```python
from build123d import *

# Parameters (mm, degrees)
F0_R     = 20
F1_DEPTH = 6
F2_R     = 13.774889
F2_R_2   = 5.493426
F3_DEPTH = 2
F4_D     = 3


with BuildPart() as f1:
    # F0 (on Front) → F1 (new body)
    with BuildSketch(Plane.XZ):
        Circle(F0_R)
    extrude(amount=F1_DEPTH)

    # F2 (on face) → F3 (cut)
    with BuildSketch(Plane.XZ.offset(6)):
        Circle(F2_R)
        Circle(F2_R_2, mode=Mode.SUBTRACT)
    extrude(amount=-F3_DEPTH, mode=Mode.SUBTRACT)

    # F4 (through all)
    with Locations(Plane.XZ.offset(6)):
        with Locations((0, 0)):
            Hole(F4_D / 2)


solid = f1.part
```
Source: CAD feature listing. Evaluate the final solid. Frame: model axes, mm. A direction names the side the tool comes from. Give positions to 0.01 mm unless a question says otherwise; leave off trailing zeros. Loops run counter-clockwise (first coordinate to the right, second up) from the corner with the lowest first, then second, coordinate; pieces in that order, holes last. Notation, with made-up numbers: (48, -16) -> (84, -16) arc R12 ccw to (84, -3) -> close; hole circle Ø10 at (2, -37). An arc over 180 degrees is marked (long way). Put each result on its own line as item: value. Start each with the question number.
1) Material intervals for probe 1 along Z at (x, y) = (0, -4.8); probe 2 along X at (y, z) = (-4.15, -5); probe 3 along Y at (x, z) = (4, -13), sorted ascending.
2) Cut plane C-C (y = -5.25). Return loops of the section in (x, z).
3) Contact query for flat-ended pins moving along their axis: P1, Ø2, axis at x = 2, y = -1, coming from the +Z side (3 decimals); P2, Ø5, axis at x = -10.5, z = 6, coming from the -Y side; P3, Ø4, axis at x = 10, z = -4.5, coming from the -Y side. Output: stop coordinate, or through.
4) Cut plane B-B (z = 0). Return loops of the section in (x, y), then the cut area to 3 significant figures.
5) Cut plane A-A (x = 0). Return loops of the section in (y, z), then the cut area to 3 significant figures.
6) Reachability of faces 4 (the face through (-5, -6, -13)), 5 (the face through (-1.79, -5.01, 13.66)) from +Z, -Z, +X, -X, +Y, -Y: full face, straight path, thin tool, end or side. Return the list, or none.
7) Cut plane D-D (y = -2.6). Return loops of the section in (x, z), then the cut area to 3 significant figures.
8) Draft query along Z for faces 1 (the face through (-4.336, -2.958, -19.524)), 2 (the face through (6, -4, 0)), 3 (the face through (-1.3, -6, -1.1)). Return one class per face: released by +Z, released by -Z, zero draft, split by the parting line, or undercut.
Results are:
1. probe 1: z = -20 to -13.77, -5.49 to -1.5, 1.5 to 5.49, 13.77 to 20
1. probe 2: x = -19.36 to -12.84, -2.28 to 2.28, 12.84 to 19.36
1. probe 3: y = -4 to 0
2. outline: circle Ø40 at (0, 0); circle Ø10.99 at (0, 0); hole circle Ø27.55 at (0, 0); hole circle Ø3 at (0, 0)
3. P1: stops at z = 19.975
3. P2: stops at y = -6
3. P3: stops at y = -4
4. outline: (-20, -6) -> (-13.77, -6) -> (-13.77, -4) -> (-5.49, -4) -> (-5.49, -6) -> (-1.5, -6) -> (-1.5, 0) -> (-20, 0) -> close; (1.5, -6) -> (5.49, -6) -> (5.49, -4) -> (13.77, -4) -> (13.77, -6) -> (20, -6) -> (20, 0) -> (1.5, 0) -> close
4. area: 189 mm2
5. outline: (-6, -20) -> (0, -20) -> (0, -1.5) -> (-6, -1.5) -> (-6, -5.49) -> (-4, -5.49) -> (-4, -13.77) -> (-6, -13.77) -> close; (-6, 1.5) -> (0, 1.5) -> (0, 20) -> (-6, 20) -> (-6, 13.77) -> (-4, 13.77) -> (-4, 5.49) -> (-6, 5.49) -> close
5. area: 189 mm2
6. face 4: +Z, -Z, +X, -X, -Y
6. face 5: -Y
7. outline: circle Ø40 at (0, 0); hole circle Ø3 at (0, 0)
7. area: 1,250 mm2
8. face 1: split by the parting line
8. face 2: undercut
8. face 3: zero draft
